The model under review builds one solid part; all positions refer to its coordinate system, in mm. Give positions to 0.01 mm unless a question says otherwise; leave off trailing zeros. Loops run counter-clockwise (first coordinate to the right, second up) from the corner with the lowest first, then second, coordinate; pieces in that order, holes last. Notation, with made-up numbers: (71, 7) -> (112, 7) arc R20 cw to (112, 32) -> close; hole circle Ø4 at (-36, -26). An arc over 180 degrees is marked (long way). Write each question's results on one line, items separated by ' | '. Start each with the question number.
Q1. Wall thickness on L1, parallel to Z at x = -18, y = 2.5; L2, parallel to Z at x = 18, y = 1.75; L3, parallel to Z at x = -39.5, y = 0.8: over which ranges is each line inside the solid? List them lowest first. Write a range as [from, to].
Q2. We need section A-A (x = -17). Write out the cut boundary in (y, z), plus the area to 3 significant figures.
Q3. Insertion check: pin 1 Ø1.8 at (x, z) = (56.5, 61.8) entering from +Y. The pin has a flat end and moves straight along its axis. Give the tip position at first contact, or say it passes through.
from build123d import *

# Parameters (mm, degrees)
SKETCH1_W           = 140
SKETCH1_H           = 148.6
BOSS_EXTRUDE1_DEPTH = 3
SKETCH2_R           = 3
SKETCH2_R_2         = 1.5
CUT_EXTRUDE1_DEPTH  = 4
FILLET1_R           = 5
CIRPATTERN1_COUNT   = 2


with BuildPart() as part:
    # Sketch1 → Boss-Extrude1 (new body)
    with BuildSketch(Plane(origin=(0, 0, 0), x_dir=(1, 0, 0), z_dir=(0, 1, 0))):
        Rectangle(SKETCH1_W, SKETCH1_H)
    extrude(amount=BOSS_EXTRUDE1_DEPTH)

    # Sketch2 → Cut-Extrude1 (cut, through all)
    with BuildSketch(Plane(origin=(0, 3, 0), x_dir=(1, 0, 0), z_dir=(0, 1, 0))):
        with Locations((-18, 26.8)):
            Circle(SKETCH2_R)
        with Locations((-18, 61.8)):
            Circle(SKETCH2_R)
        with Locations((-1, 61.8)):
            Circle(SKETCH2_R_2)
        with Locations((-1, 26.8)):
            Circle(SKETCH2_R_2)
        with Locations((-56.5, 61.8)):
            Circle(SKETCH2_R_2)
        with Locations((-39.5, -8.2)):
            Circle(SKETCH2_R_2)
    cut_extrude1 = extrude(amount=-CUT_EXTRUDE1_DEPTH, mode=Mode.SUBTRACT)

    # Fillet1
    fillet1_edges = [part.edges().sort_by_distance(p)[0] for p in [
        (-70, 1.5, -74.3),
        (70, 1.5, -74.3),
        (70, 1.5, 74.3),
        (-70, 1.5, 74.3),
    ]]
    fillet(fillet1_edges, radius=FILLET1_R)

    # CirPattern1: Cut-Extrude1 ×2 about axis
    cirpattern1_axis = Axis((0, 0, 0), (0, 1, 0))
    for i in range(1, CIRPATTERN1_COUNT):
        add(cut_extrude1.rotate(cirpattern1_axis, i * 360 / CIRPATTERN1_COUNT), mode=Mode.SUBTRACT)


solid = part.part
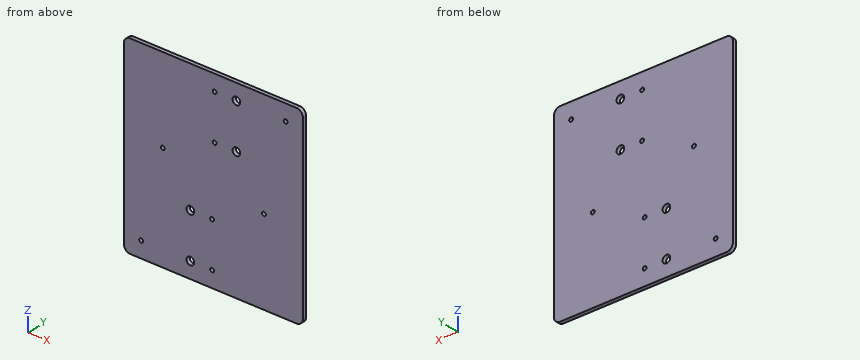
Output:
1) L1: [-74.3, -64.8], [-58.8, -29.8], [-23.8, 74.3] | L2: [-74.3, 23.8], [29.8, 58.8], [64.8, 74.3] | L3: [-74.3, 6.7], [9.7, 74.3]
2) outline: (0, -74.3) -> (3, -74.3) -> (3, -64.63) -> (0, -64.63) -> close; (0, -58.97) -> (3, -58.97) -> (3, -29.63) -> (0, -29.63) -> close; (0, -23.97) -> (3, -23.97) -> (3, 74.3) -> (0, 74.3) -> close | area: 412 mm2
3) pin 1: through
